Autodesk Inventor part; units mm, degrees
ref_plane "YZ Plane" through (0, 0, 0) normal (1, 0, 0) x (0, 1, 0)
ref_plane "XZ Plane" through (0, 0, 0) normal (0, 1, 0) x (-1, 0, 0)
ref_plane "XY Plane" through (0, 0, 0) normal (0, 0, 1) x (1, 0, 0)
ref_plane "작업 평면1" through (0, -41, 8.5) normal (0, 0, 1) x (1, 0, 0)
sketch "스케치1" plane through (0, -41, 8.5) normal (0, 0, 1) x (1, 0, 0)
  circle A0 centre (0, -40.5) radius 15
  circle A1 centre (0, -40.5) radius 5
  circle A2 centre (0, -40.5) radius 14.8
  circle A3 centre (0, -40.5) radius 5.3
  circle A4 centre (0, -40.5) radius 13.1
  circle A5 centre (0, -40.5) radius 7
  point P0 (0, 41)
  dimension "d0" = 0.2
  dimension "d1" = 0.3
  dimension "d2" = 1.7
  dimension "d3" = 1.7
extrude "돌출1" add sketch "스케치1" along normal mid plane 9 contours A2
ref_plane "작업 평면2" through (0, -81.5, 8.5) normal (0, 0, 1) x (1, 0, 0)
sketch "스케치3" plane through (0, -81.5, 13) normal (0, 0, 1) x (1, 0, 0)
  circle A0 centre (0, 0) radius 13.1
  circle A1 centre (0, 0) radius 7.8
  point P0 (0, 81.5)
  dimension "d11" = 5.3
extrude "돌출2" add sketch "스케치3" against normal up to surface (9 mm away)
sketch "스케치6" plane through (0, 0, 0) normal (1, 0, 0) x (0, 1, 0)
  line L0 (-96.3, 4) -> (-66.7, 4)
  line L1 (-66.7, 13) -> (-96.3, 13)
  line L2 (-66.7, 4) -> (-66.7, 13)
  line L3 (-96.3, 4) -> (-96.3, 13)
  circle A0 centre (-72.1, 8.5) radius 3.2
  line L4 (-81.5, -2.6) -> (-81.5, 15.6)
  line L5 (-68.9, 15.8649) -> (-68.9, 0.3346)
  circle A1 centre (-72.1, 8.5) radius 2.8 construction
  line L6 (-74.9, 15.3235) -> (-74.9, 0.5874) construction
  circle A2 centre (-71.7, 8.5) radius 2.8 construction
  line L7 (-74.5, 4.469) -> (-74.5, 12.0599) construction
  point P0 (0, 0)
  dimension "d19" = 6.4
  dimension "d21" = 4.5
  dimension "d22" = 29.6
  dimension "d23" = 2.2
  dimension "d25" = 5.6
  dimension "d26" = 5.6
revolve "회전2" cut sketch "스케치6" angle 360 about axis through (0, -81.5, 8.5) along (0, 0, 1) contours A0
properties part number "custom_bearing" material "고무, 검은색"
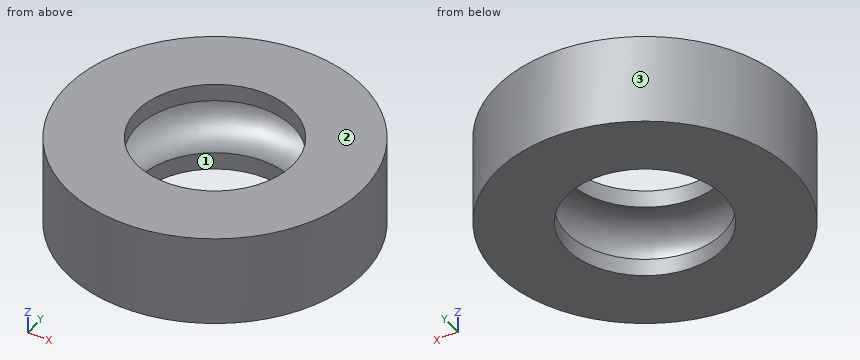
The listing builds one solid part. Answer for the finished solid, in the listing's coordinates (mm). Face numbers are marked on the shaded views. Coordinates: 2 decimals unless noted, no trailing zeros. Loops run counter-clockwise (first coordinate to the right, second up) from the corner with the lowest first, then second, coordinate; pieces in that order, holes last. Notation, with made-up numbers: (24.25, 15.25) -> (50.25, 15.25) arc R34 cw to (50.25, 47.25) -> close; hole circle Ø7 at (66, 31.5). An arc over 180 degrees is marked (long way). Answer in a Markdown table with one row per item. Add a question column.
1. Consider line 1 (Y direction, x = 0, z = 4.4); line 2 (Y direction, x = -0.75, z = 7.25); line 3 (Z direction, x = -4.25, y = -89.5). Determine where each line is inside the solid, lowest interval first. Write a range as [from, to].
2. Determine the mould class of the marked faces 1, 2 and 3 for opening direction X: +X half, -X half, draft (parallel to the pull), parting line (faces both ways), or undercut.
3. The part is cut by section C-C, the plane z = 9.5. Write down the section's boundary in (x, y), then the cut area to 3 significant figures.
4. The part is cut by section A-A, the plane x = 0. Write down the section's boundary in (y, z), then the cut area to 3 significant figures.
5. The part is cut by section B-B, the plane y = -81.5. Write down the section's boundary in (x, z).
6. The part is cut by section D-D, the plane z = 6.5. Write down the section's boundary in (x, y), then the cut area to 3 significant figures.
7. Flat-ended cylindrical pins translate along their axes: P1, Ø1.5, axis at y = -75.5, z = 5, coming from the -X side; P2, Ø1, axis at x = 2, z = 9, coming from the -Y side; P3, Ø1, axis at x = -6.5, z = 9, coming from the +Y side. Find the tip coordinate at first contact, or state that the pin passes through.
Answer below:
| question | item | result |
|---|---|---|
| 1 | line 1 | [-96.3, -89.3], [-73.7, -66.7] |
| 1 | line 2 | [-96.28, -93.82], [-69.18, -66.72] |
| 1 | line 3 | [4, 5.32], [11.68, 13] |
| 2 | face 1 | undercut |
| 2 | face 2 | draft |
| 2 | face 3 | parting line |
| 3 | outline | circle Ø29.6 at (0, -81.5); hole circle Ø24.88 at (0, -81.5) |
| 3 | area | 202 mm2 |
| 4 | outline | (-96.3, 4) -> (-89.3, 4) -> (-89.3, 5.73) arc R3.2 cw (long way) to (-89.3, 11.27) -> (-89.3, 13) -> (-96.3, 13) -> close; (-73.7, 4) -> (-66.7, 4) -> (-66.7, 13) -> (-73.7, 13) -> (-73.7, 11.27) arc R3.2 cw (long way) to (-73.7, 5.73) -> close |
| 4 | area | 74.2 mm2 |
| 5 | outline | (-14.8, 4) -> (-7.8, 4) -> (-7.8, 5.73) arc R3.2 cw (long way) to (-7.8, 11.27) -> (-7.8, 13) -> (-14.8, 13) -> close; (7.8, 4) -> (14.8, 4) -> (14.8, 13) -> (7.8, 13) -> (7.8, 11.27) arc R3.2 cw (long way) to (7.8, 5.73) -> close |
| 6 | outline | circle Ø29.6 at (0, -81.5); hole circle Ø23.8 at (0, -81.5) |
| 6 | area | 243 mm2 |
| 7 | P1 | x = -13.84 |
| 7 | P2 | y = -96.22 |
| 7 | P3 | y = -67.97 |
